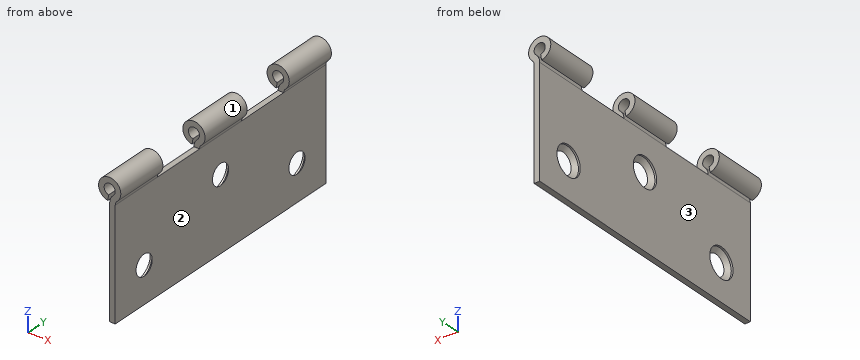
```python
from build123d import *

# Parameters (mm, degrees)
BOSS_EXTRUDE1_DEPTH                       = 38.1
SKETCH3_W                                 = 6.724757914
SKETCH3_H                                 = 15.24
CUT_EXTRUDE1_DEPTH                        = 4.175
CUT_EXTRUDE1_DEPTH_BACK                   = 4.175
CSK_FOR_8_FLAT_HEAD_MACHINE_SCREW_2_COUNT = 2
CSK_FOR_8_FLAT_HEAD_MACHINE_SCREW_2_PITCH = 29.553945574
CSK_FOR_8_FLAT_HEAD_MACHINE_SCREW_3_COUNT = 2
CSK_FOR_8_FLAT_HEAD_MACHINE_SCREW_3_PITCH = 55.283171943


with BuildPart() as part:
    # Sketch2 → Boss-Extrude1 (new body, symmetric)
    with BuildSketch(Plane(origin=(0, 0, 0), x_dir=(1, 0, 0), z_dir=(0, 1, 0))):
        with BuildLine():
            Line((1.5875, 34.925), (0, 34.925))
            Line((0, 34.925), (0, 3.549757914))
            ThreePointArc((0, 3.549757914), (0.2766348, 2.253569592), (1.058333333, 1.183252638))
            ThreePointArc((1.058333333, 1.183252638), (-0.435047689, -1.526725175), (-0.275666482, 1.563382308))
            Line((-0.275666482, 1.563382308), (-0.551332964, 3.126764616))
            ThreePointArc((-0.551332964, 3.126764616), (-0.870095378, -3.053450349), (2.116666667, 2.366505276))
            ThreePointArc((2.116666667, 2.366505276), (1.7258174, 2.901663753), (1.5875, 3.549757914))
            Line((1.5875, 3.549757914), (1.5875, 34.925))
        make_face()
    extrude(amount=BOSS_EXTRUDE1_DEPTH, both=True)

    # Sketch3 → Cut-Extrude1 (cut, two sides)
    with BuildSketch(Plane(origin=(0, 0, 0), x_dir=(0, 0, -1), z_dir=(1, 0, 0))) as cut_extrude1_sk:
        with Locations((0.187378957, 15.24)):
            Rectangle(SKETCH3_W, SKETCH3_H)
        with Locations((0.187378957, -15.24)):
            Rectangle(SKETCH3_W, SKETCH3_H)
    extrude(amount=CUT_EXTRUDE1_DEPTH, mode=Mode.SUBTRACT)
    extrude(cut_extrude1_sk.sketch, amount=-CUT_EXTRUDE1_DEPTH_BACK, mode=Mode.SUBTRACT)

    # Sketch4 → CSK for #8 Flat Head Machine Screw (100)1 (revolve, cut)
    with BuildSketch(Plane(origin=(0, -27.641585971, -24.466585971), x_dir=(0, 0, 1), z_dir=(0, 1, 0))):
        Polygon((0, 0), (0, 3.175), (2.2479, 3.175), (2.2479, 2.159767624), (4.2164, 0.508), (4.2164, 0), align=None)
    csk_for_8_flat_head_machine_screw_100 = revolve(axis=Axis((-6.35, -27.641585971, -24.466585971), (1, 0, 0)), mode=Mode.SUBTRACT)

    # CSK for _8 Flat Head Machine Screw _ 2: CSK for #8 Flat Head Machine Screw (100)1 ×2
    with Locations(*[Vector(0, 0.935292579, 0.35387539) * (i * CSK_FOR_8_FLAT_HEAD_MACHINE_SCREW_2_PITCH) for i in range(1, CSK_FOR_8_FLAT_HEAD_MACHINE_SCREW_2_COUNT)]):
        add(csk_for_8_flat_head_machine_screw_100, mode=Mode.SUBTRACT)

    # CSK for _8 Flat Head Machine Screw _ 3: CSK for #8 Flat Head Machine Screw (100)1 ×2
    with Locations(*[(0, i * CSK_FOR_8_FLAT_HEAD_MACHINE_SCREW_3_PITCH, 0) for i in range(1, CSK_FOR_8_FLAT_HEAD_MACHINE_SCREW_3_COUNT)]):
        add(csk_for_8_flat_head_machine_screw_100, mode=Mode.SUBTRACT)


solid = part.part
```
Source: CAD feature listing. Evaluate the final solid. Frame: model axes, mm. Face numbers are marked on the shaded views. A direction names the side the tool comes from. Give positions to 0.01 mm unless a question says otherwise; leave off trailing zeros. Loops run counter-clockwise (first coordinate to the right, second up) from the corner with the lowest first, then second, coordinate; pieces in that order, holes last. Notation, with made-up numbers: (29.25, 77.5) -> (60.25, 77.5) arc R21 cw to (60.25, 89.5) -> close; hole circle Ø9 at (17, 5). An arc over 180 degrees is marked (long way). Use a Markdown table: item, result. Add a question column.
(1) Section query A-A (z = 0). Output: boundary loops of the cut face in (x, y) (1 decimal), then the cut area to 3 significant figures.
(2) Access query for the marked faces 1, 2 and 3. Directions: +Z, -Z, +X, -X, +Y, -Y. A direction counts if a zero-diameter tool reaches every point of the face in a straight line with its end or side. Return the directions, or none.
(3) Ray query, line 1 (X direction, y = 31.5, z = 0) (1 decimal); line 2 (Z direction, x = 1.25, y = -11.5) (3 decimals); line 3 (X direction, y = -22, z = -20). Return the intervals inside material, ascending.
(4) First-contact query: pin 1 Ø12 at (y, z) = (-1.5, -8.5) entering from +X; pin 2 Ø8 at (y, z) = (-17.5, -3.5) entering from +X; pin 3 Ø1.5 at (y, z) = (8.5, -24.5) entering from -X; pin 4 Ø5 at (y, z) = (-27.64, -24.47) entering from +X. Flat tips, straight axial feed; report the tip coordinate or a pass-through.
(5) Section query C-C (y = -14). Output: boundary loops of the cut face in (x, z) (1 decimal).
(6) Section query D-D (z = -31). Output: boundary loops of the cut face in (x, y).
Checked values:
| question | item | result |
|---|---|---|
| 1 | outline | (-3.2, -38.1) -> (-1.6, -38.1) -> (-1.6, -22.9) -> (-3.2, -22.9) -> close; (-3.2, -7.6) -> (-1.6, -7.6) -> (-1.6, 7.6) -> (-3.2, 7.6) -> close; (-3.2, 22.9) -> (-1.6, 22.9) -> (-1.6, 38.1) -> (-3.2, 38.1) -> close; (1.6, -38.1) -> (3.2, -38.1) -> (3.2, -22.9) -> (1.6, -22.9) -> close; (1.6, -7.6) -> (3.2, -7.6) -> (3.2, 7.6) -> (1.6, 7.6) -> close; (1.6, 22.9) -> (3.2, 22.9) -> (3.2, 38.1) -> (1.6, 38.1) -> close |
| 1 | area | 145 mm^2 |
| 2 | face 1 | +Y, -Y |
| 2 | face 2 | -Z, +X, +Y, -Y |
| 2 | face 3 | -Z, -X, +Y, -Y |
| 3 | line 1 | -3.2 to -1.6, 1.6 to 3.2 |
| 3 | line 2 | -34.925 to -3.55 |
| 3 | line 3 | 0 to 1.59 |
| 4 | pin 1 | x = 1.98 |
| 4 | pin 2 | x = 1.59 |
| 4 | pin 3 | x = 0 |
| 4 | pin 4 | through |
| 5 | outline | (0, -34.9) -> (1.6, -34.9) -> (1.6, -3.5) -> (0, -3.5) -> close |
| 6 | outline | (0, -38.1) -> (1.59, -38.1) -> (1.59, 38.1) -> (0, 38.1) -> close |
